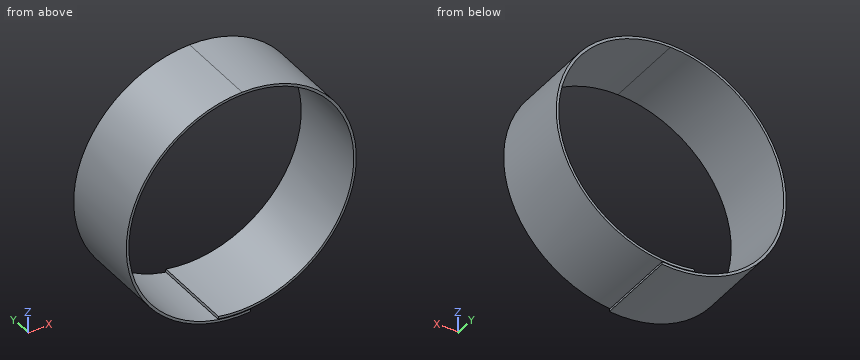
from build123d import *

# Parameters (mm, degrees)
BASE_FLANGE1_DEPTH = 25


# Sheet-metal steps are written as plain solids
with BuildPart() as part:
    # Sketch1 → Base-Flange1 (new body)
    with BuildSketch(Plane(origin=(0, 0, 0), x_dir=(1, 0, 0), z_dir=(0, 1, 0))):
        with BuildLine():
            ThreePointArc((2.605767321, 35.404236705), (-35.476051098, 1.303763201), (0, -35.5))
            ThreePointArc((0, -35.5), (34.801944096, 3.21815642), (-7.394232679, 33.710017876))
            Line((-7.394232679, 33.710017876), (-7.563243712, 34.491961142))
            ThreePointArc((-7.563243712, 34.491961142), (35.597417103, 3.303142853), (0, -36.3))
            ThreePointArc((0, -36.3), (-36.275511405, 1.33314378), (2.664488838, 36.202078659))
            Line((2.664488838, 36.202078659), (2.605767321, 35.404236705))
        make_face()
    extrude(amount=BASE_FLANGE1_DEPTH)


solid = part.part
Check sheet for the modelled part. Datum: model origin and axes. Units: mm. Round coordinates to 2 decimals unless told otherwise and drop trailing zeros. Loops run counter-clockwise (first coordinate to the right, second up) from the corner with the lowest first, then second, coordinate; pieces in that order, holes last. Notation, with made-up numbers: (19.5, 75) -> (38.5, 75) arc R23 ccw to (38.5, 110) -> close; hole circle Ø9 at (24.5, 72.25). An arc over 180 degrees is marked (long way). Put each result on its own line as item: value. Start each with the question number.
1. Section check A-A (x = 0). Enter the section's corners in (y, z), plus the area to 3 significant figures.
2. Scan lines: probe 1 along Z at (x, y) = (0, 16.75); probe 2 along X at (y, z) = (10, 0.5); probe 3 along Z at (x, y) = (-4, 12.5). Record each from-to range of solid material in increasing order.
3. Section check D-D (x = -26). Enter the section's corners in (y, z), plus the area to 3 significant figures.
4. Section check C-C (y = 6). Enter the section's corners in (x, z).
5. Section check B-B (z = 27). Enter the section's corners in (x, y), plus the area to 3 significant figures.
6. Gauge pin test, flat ends, axial feed: pin 1 (8 mm diameter, centred on x = -11.5, y = 22.5, fed in from +Z); pin 2 (10 mm diameter, centred on y = 15.5, z = -13, fed in from -X); pin 3 (3 mm diameter, centred on x = -1, y = 15, fed in from -Z). Record the tip position at first contact, or that the pin passes through.
Findings:
1. outline: (0, -36.3) -> (25, -36.3) -> (25, -35.5) -> (0, -35.5) -> close; (0, -35.3) -> (25, -35.3) -> (25, -34.5) -> (0, -34.5) -> close; (0, 35.5) -> (25, 35.5) -> (25, 36.3) -> (0, 36.3) -> close
1. area: 60.0 mm^2
2. probe 1: z = -36.3 to -35.5, -35.3 to -34.5, 35.5 to 36.3
2. probe 2: x = -36.3 to -35.5, 35 to 35.8
2. probe 3: z = -36.08 to -35.27, -35.08 to -34.27, 35.27 to 36.08
3. outline: (0, -25.33) -> (25, -25.33) -> (25, -24.17) -> (0, -24.17) -> close; (0, 24.17) -> (25, 24.17) -> (25, 25.33) -> (0, 25.33) -> close
3. area: 58.0 mm^2
4. outline: (-7.56, -34.49) arc R35.8 ccw (long way) to (0, 36.3) arc R36.3 ccw (long way) to (2.66, -36.2) -> (2.61, -35.4) arc R35.5 cw (long way) to (0, 35.5) arc R35 cw (long way) to (-7.39, -33.71) -> close
5. outline: (-24.26, 0) -> (-23.05, 0) -> (-23.05, 25) -> (-24.26, 25) -> close; (22.86, 0) -> (24.07, 0) -> (24.07, 25) -> (22.86, 25) -> close
5. area: 60.5 mm^2
6. pin 1: stops at z = 35.52
6. pin 2: stops at x = -35.41
6. pin 3: stops at z = -36.3
